Job drawing, mm, ordinate dimensions from the low corner. One solid piece. Round coordinates to 2 decimals unless told otherwise and drop trailing zeros. Order: outer loops, then holes, each group sorted by start corner. A loop starts at its lowest first (then second) coordinate and runs counter-clockwise, first axis right, second up. Notation, with made-up numbers: (8.5, 15.5) -> (63.5, 15.5) arc R7 ccw to (63.5, 26.5) -> close; hole circle Ø2 at (-9, -8.75). An arc over 180 degrees is marked (long way). Return JSON: item names as keys, results as strings. Group by question number.
Q1. Cut at C-C (z = 2.75). Write the cut outline in (x, y) (3 decimals).
Q2. Probe line 1 along Y through (x, z) = (9.1, 5) (3 decimals); line 2 along Y through (x, z) = (10.25, 5.5); line 3 along Z through (x, y) = (14.5, 5.5). List the from-to ranges inside material, lowest first.
Q3. Cut at D-D (z = 5.75). Write the cut outline in (x, y) (3 decimals), then the cut area to 4 significant figures.
Q4. Mould opens along X. For the marked faces 1, 2 and 3 say: +X half, -X half, draft (parallel to the pull), parting line (faces both ways), or undercut.
Q5. Cut at A-A (x = 9.1). Write the cut outline in (y, z) (3 decimals).
Q6. Flat gauge pin, fed straight in: pin 1 (10 mm diameter, centred on x = 16, y = 15.5, fed in from -Z). Where does the tip first touch, or does it go through?
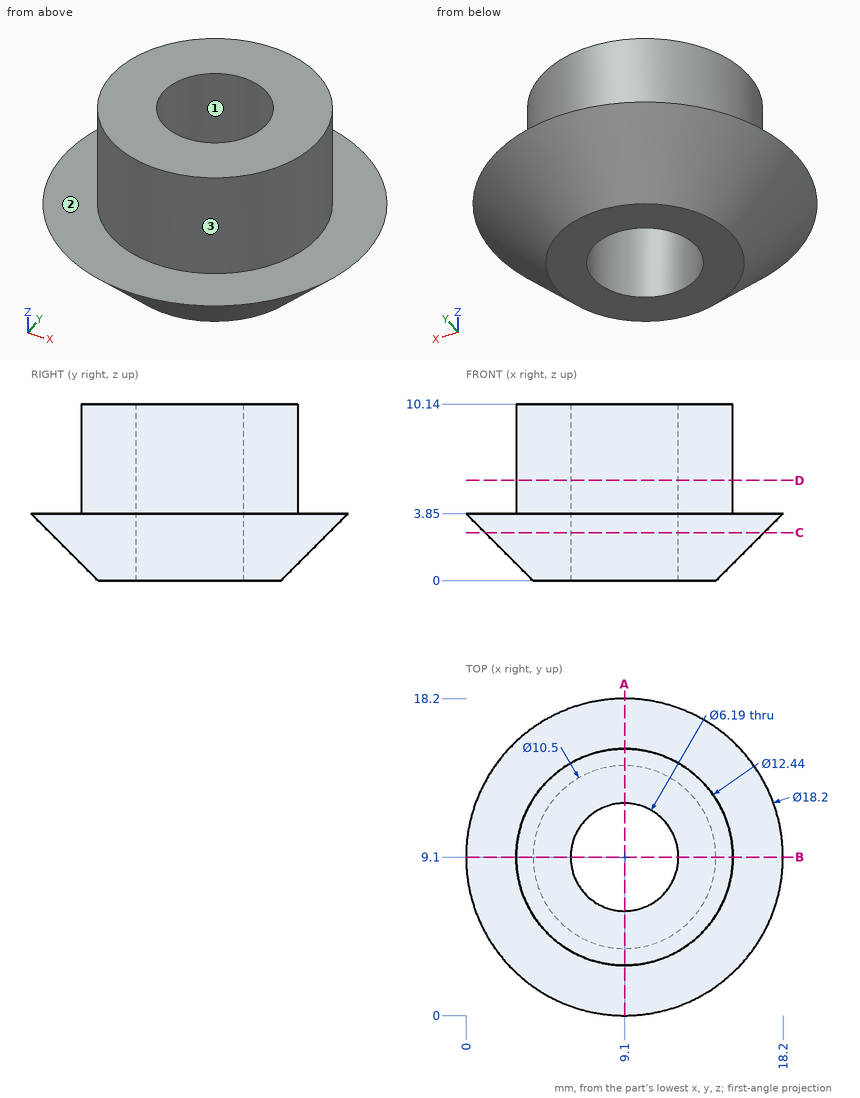
Solution:
{
 "1": {"outline": "circle Ø16 at (9.1, 9.1); hole circle Ø6.19 at (9.1, 9.1)"},
 "2": {"line 1": "y = 2.88 to 6.005, 12.195 to 15.32", "line 2": "y = 2.99 to 6.23, 11.97 to 15.21", "line 3": "z = 1.24 to 3.85"},
 "3": {"outline": "circle Ø12.44 at (9.1, 9.1); hole circle Ø6.19 at (9.1, 9.1)", "area": "91.45 mm²"},
 "4": {"face 1": "undercut", "face 2": "draft", "face 3": "parting line"},
 "5": {"outline": "(0, 3.85) -> (3.85, 0) -> (6.005, 0) -> (6.005, 10.14) -> (2.88, 10.14) -> (2.88, 3.85) -> close; (12.195, 0) -> (14.35, 0) -> (18.2, 3.85) -> (15.32, 3.85) -> (15.32, 10.14) -> (12.195, 10.14) -> close"},
 "6": {"pin 1": "stops at z = 0"}
}
